Verification items for this drawing (mm, ordinates from the low corner). A direction names the side the tool comes from. Round coordinates to 2 decimals unless told otherwise and drop trailing zeros. Write each loop counter-clockwise with the first axis right and the second up, starting at its lowest first coordinate (ties: lowest second). Pieces come first, ordered by that corner, then holes. Notation, with made-up numbers: (-34.5, 37) -> (-0.5, 37) arc R21 cw to (-0.5, 55) -> close; hole circle Ø4 at (45.5, 82). An arc over 180 degrees is marked (long way). One line per question, with ' | ' between items.
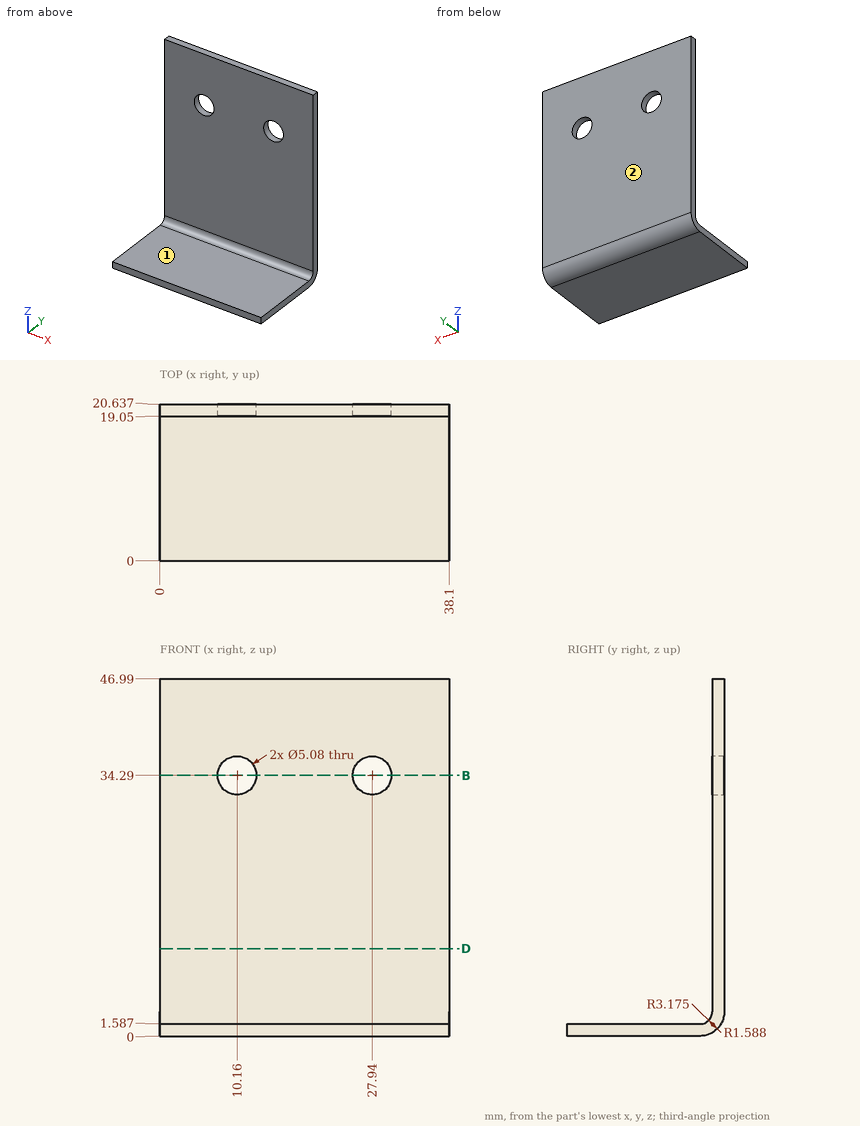
(1) Sectioned sample at B-B on z = 34.29. Record the cut outline in (x, y).
Resolved:
outline: (0, 19.05) -> (7.62, 19.05) -> (7.62, 20.64) -> (0, 20.64) -> close; (12.7, 19.05) -> (25.4, 19.05) -> (25.4, 20.64) -> (12.7, 20.64) -> close; (30.48, 19.05) -> (38.1, 19.05) -> (38.1, 20.64) -> (30.48, 20.64) -> close
(2) Material ranges on line 1 (X direction, y = 20.25, z = 34.29); line 2 (Y direction, x = 13, z = 32); line 3 (Z direction, x = 14, y = 15.5), recorded low to high.
Resolved:
line 1: x = 0 to 7.62, 12.7 to 25.4, 30.48 to 38.1 | line 2: y = 19.05 to 20.64 | line 3: z = 0 to 1.59
(3) Go/stop test with flat-tipped pins: pin 1 (12 mm diameter, centred on x = 8, y = 10, fed in from +Z); pin 2 (8 mm diameter, centred on x = 27.94, z = 34.29, fed in from -Y); pin 3 (8 mm diameter, centred on x = 25.5, z = 6.5, fed in from -Y). Record where each tip stops, or that it passes through.
Resolved:
pin 1: stops at z = 1.59 | pin 2: stops at y = 19.05 | pin 3: stops at y = 18.9
(4) Access from +Z, -Z, +X, -X, +Y, -Y to the whole of each face (thin tool, end or side, straight path). Record for the marked faces 1 and 2.
Resolved:
face 1: +Z, +X, -X, -Y | face 2: +Z, -Z, +X, -X, +Y
(5) Sectioned sample at D-D on z = 11.5. Record the cut outline in (x, y).
Resolved:
outline: (0, 19.05) -> (38.1, 19.05) -> (38.1, 20.64) -> (0, 20.64) -> close
